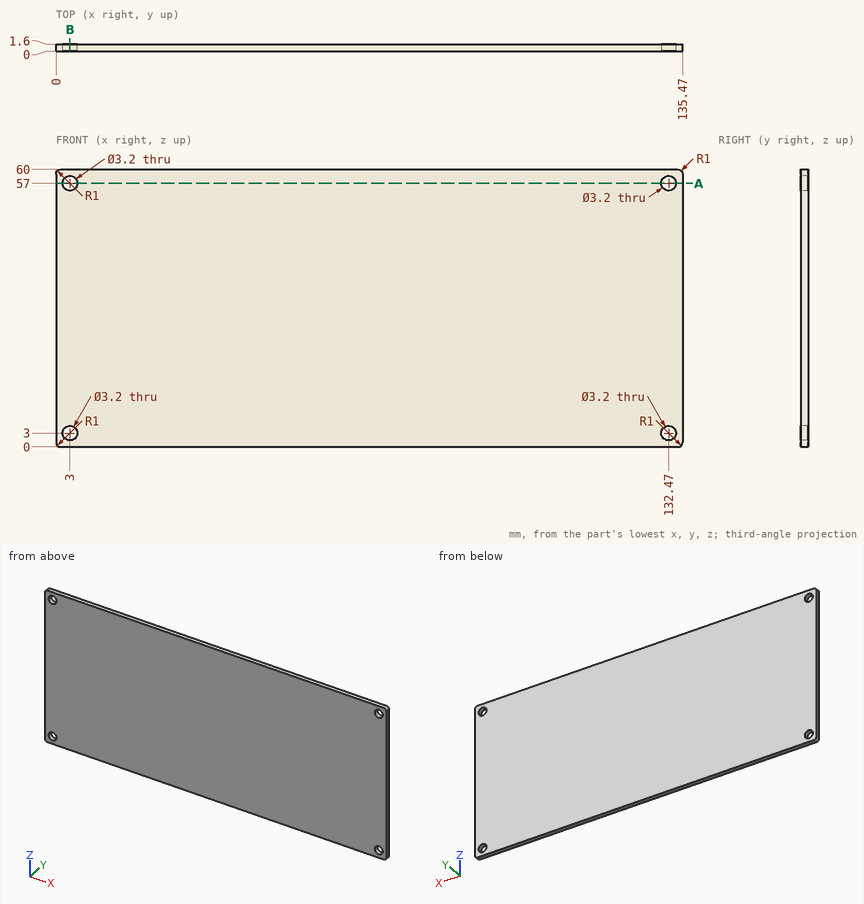
The figure shows three views and two pictorial views of one solid part (mm, origin at its lowest corner). Answer the questions. Round coordinates to 2 decimals unless told otherwise and drop trailing zeros. Order: outer loops, then holes, each group sorted by start corner. A loop starts at its lowest first (then second) coordinate and runs counter-clockwise, first axis right, second up.
Q1. A cutting plane is placed at A-A, the plane z = 57. Determine the outline of the cut face in (x, y), then the cut area to 3 significant figures.
Solution:
outline: (0, 0) - (1.4, 0) - (1.4, 1.6) - (0, 1.6) - close; (4.6, 0) - (130.87, 0) - (130.87, 1.6) - (4.6, 1.6) - close; (134.07, 0) - (135.47, 0) - (135.47, 1.6) - (134.07, 1.6) - close
area: 207 mm2
Q2. Find the intervals of material crossed by line 1 along Z through (x, y) = (132.47, 0.85); line 2 along X through (y, z) = (0.8, 57); line 3 along X through (y, z) = (0.85, 57.5), in increasing order.
Solution:
line 1: z = 0 to 1.4, 4.6 to 55.4, 58.6 to 60
line 2: x = 0 to 1.4, 4.6 to 130.87, 134.07 to 135.47
line 3: x = 0 to 1.48, 4.52 to 130.95, 133.99 to 135.47
Q3. Given pin 1 Ø1.9 at (x, z) = (3, 3) entering from +Y (1 decimal), flat-ended and moving along its own axis, determine where the tip first touches the part or whether it passes through.
Solution:
pin 1: passes through
Q4. A cutting plane is placed at B-B, the plane x = 3. Determine the outline of the cut face in (y, z).
Solution:
outline: (0, 0) - (1.6, 0) - (1.6, 1.4) - (0, 1.4) - close; (0, 4.6) - (1.6, 4.6) - (1.6, 55.4) - (0, 55.4) - close; (0, 58.6) - (1.6, 58.6) - (1.6, 60) - (0, 60) - close
